Here's how the part is built. I have some questions about the finished solid (model axes, mm). A direction names the side the tool comes from. Round coordinates to 2 decimals unless told otherwise and drop trailing zeros. Loops run counter-clockwise (first coordinate to the right, second up) from the corner with the lowest first, then second, coordinate; pieces in that order, holes last. Notation, with made-up numbers: (-18, -31) -> (39, -31) arc R27 ccw to (39, -4) -> close; hole circle Ø5 at (13.5, -27.75). An arc over 180 degrees is marked (long way). Use one line per item in the form item = value. Start each with the question number.
Item 1: I'm going to push flat-ended pins straight in: pin 1 Ø4 at (x, y) = (1, 1) entering from -Z; pin 2 Ø0.8 at (x, z) = (-13.5, -4) entering from -Y; pin 3 Ø0.5 at (y, z) = (-2.5, -5) entering from +X. Where does each tip first touch, or does it pass through?
Item 2: Thinking about a two-plate mould opening in Y: for faces 1 (the face through (2, 9, -1)), 2 (the face through (-2.3, 9.7, 0)), 3 (the face through (-13.5, -8.1, -4.7)), 4 (the face through (-13.5, -7.1, -4.7)), which applies, released by +Y, released by -Y, zero draft, split by the parting line, or undercut?
Item 3: If we section it at B-B (x = -10): Write out the boundary of the cut face in (y, z), then the cut area to 3 significant figures.
Item 4: If we section it at D-D (z = -1.25): Write out the boundary of the cut face in (x, y).
Item 5: For faces 5 (the face through (-15, -2, -1)), 6 (the face through (-12, -4, -1)), 7 (the face through (-14, -2.6, -4.7)), which set-ups out of +Z, -Z, +X, -X, +Y, -Y let a thin tool reach every point of the face, with its end or its side?
Item 6: If I drill on L1, parallel to Y at x = -13.5, z = -6.5; L2, parallel to X at y = 1.5, z = -0.5; L3, parallel to Y at x = -3.75, z = 4.25, over which ranges is the centre line in solid material (lowest first)? Write a range as [from, to].
Item 7: If we section it at C-C (y = -4.5): Write out the boundary of the cut face in (x, z).
Item 8: If we section it at A-A (z = -4): Write out the boundary of the cut face in (x, y), then the cut area to 3 significant figures.
```python
from build123d import *

# Parameters (mm, degrees)
SKETCH1_W           = 30
SKETCH1_H           = 20
BOSS_EXTRUDE1_DEPTH = 1
SKETCH2_W           = 3
SKETCH2_H           = 12.8
BOSS_EXTRUDE2_DEPTH = 2.2
SKETCH3_W           = 1
SKETCH3_H           = 1
BOSS_EXTRUDE3_DEPTH = 5
LPATTERN1_COUNT     = 6
LPATTERN1_PITCH     = 2
SKETCH4_W           = 25
SKETCH4_H           = 18
BOSS_EXTRUDE4_DEPTH = 2.6
SKETCH5_W           = 18.6
SKETCH5_H           = 18.6
BOSS_EXTRUDE5_DEPTH = 4.9


with BuildPart() as part:
    # Sketch1 → Boss-Extrude1 (new body)
    with BuildSketch(Plane.XY):
        Rectangle(SKETCH1_W, SKETCH1_H)
    extrude(amount=BOSS_EXTRUDE1_DEPTH)

    # Sketch2 → Boss-Extrude2 (add)
    with BuildSketch(Plane(origin=(0, 0, 0), x_dir=(-1, 0, 0), z_dir=(0, 0, -1))):
        with Locations((13.5, -3.6)):
            Rectangle(SKETCH2_W, SKETCH2_H)
    extrude(amount=BOSS_EXTRUDE2_DEPTH)

    # Sketch3 → Boss-Extrude3 (add)
    with BuildSketch(Plane(origin=(0, 0, -2.2), x_dir=(-1, 0, 0), z_dir=(0, 0, -1))):
        with Locations((13.5, -8.6)):
            Rectangle(SKETCH3_W, SKETCH3_H)
    boss_extrude3 = extrude(amount=BOSS_EXTRUDE3_DEPTH)

    # LPattern1: Boss-Extrude3 ×6
    with Locations(*[(0, i * LPATTERN1_PITCH, 0) for i in range(1, LPATTERN1_COUNT)]):
        add(boss_extrude3)

    # Sketch4 → Boss-Extrude4 (add)
    with BuildSketch(Plane(origin=(0, 0, 0), x_dir=(-1, 0, 0), z_dir=(0, 0, -1))):
        with Locations((-1.5, 0)):
            Rectangle(SKETCH4_W, SKETCH4_H)
    extrude(amount=BOSS_EXTRUDE4_DEPTH)

    # Sketch5 → Boss-Extrude5 (add)
    with BuildSketch(Plane.XY.offset(1)):
        with Locations((4.7, 0)):
            Rectangle(SKETCH5_W, SKETCH5_H)
    extrude(amount=BOSS_EXTRUDE5_DEPTH)


solid = part.part
```
Values found:
q1.pin_1 = -2.6
q1.pin_2 = -9.1
q1.pin_3 = -13
q2.face_1 = released by +Y
q2.face_2 = zero draft
q2.face_3 = undercut
q2.face_4 = undercut
q3.outline = (-10, 0) -> (-9, 0) -> (-9, -2.6) -> (9, -2.6) -> (9, 0) -> (10, 0) -> (10, 1) -> (-10, 1) -> close
q3.area = 66.8 mm2
q4.outline = (-15, -10) -> (-12, -10) -> (-12, 2.8) -> (-15, 2.8) -> close; (-11, -9) -> (14, -9) -> (14, 9) -> (-11, 9) -> close
q5.face_5 = +Z, -Z, -X, +Y, -Y
q5.face_6 = -Z, +Y, -Y
q5.face_7 = -Z, -X, +Y, -Y
q6.L1 = [-9.1, -8.1], [-7.1, -6.1], [-5.1, -4.1], [-3.1, -2.1], [-1.1, -0.1], [0.9, 1.9]
q6.L2 = [-15, -12], [-11, 14]
q6.L3 = [-9.3, 9.3]
q7.outline = (-15, -2.2) -> (-14, -2.2) -> (-14, -7.2) -> (-13, -7.2) -> (-13, -2.2) -> (-12, -2.2) -> (-12, 0) -> (-11, 0) -> (-11, -2.6) -> (14, -2.6) -> (14, 0) -> (15, 0) -> (15, 1) -> (14, 1) -> (14, 5.9) -> (-4.6, 5.9) -> (-4.6, 1) -> (-15, 1) -> close
q8.outline = (-14, -9.1) -> (-13, -9.1) -> (-13, -8.1) -> (-14, -8.1) -> close; (-14, -7.1) -> (-13, -7.1) -> (-13, -6.1) -> (-14, -6.1) -> close; (-14, -5.1) -> (-13, -5.1) -> (-13, -4.1) -> (-14, -4.1) -> close; (-14, -3.1) -> (-13, -3.1) -> (-13, -2.1) -> (-14, -2.1) -> close; (-14, -1.1) -> (-13, -1.1) -> (-13, -0.1) -> (-14, -0.1) -> close; (-14, 0.9) -> (-13, 0.9) -> (-13, 1.9) -> (-14, 1.9) -> close
q8.area = 6.00 mm2
